from build123d import *

# Parameters (mm, degrees)
SKICA1_R                     = 15
P_IDAT_VYSUNUT_M1_DEPTH      = 2.5
SKICA1_3_R                   = 15
P_IDAT_VYSUNUT_M2_DEPTH      = 25
P_IDAT_VYSUNUT_M2_DEPTH_BACK = 5


with BuildPart() as part:
    # Skica1 → P_idat vysunut_m1 (new body, symmetric)
    with BuildSketch(Plane.XY):
        with BuildLine():
            Line((5, 30.562589032), (5, 5))
            Line((5, 5), (32.5, 5))
            Line((32.5, 5), (32.5, -5))
            Line((32.5, -5), (-32.5, -5))
            Line((-32.5, -5), (-32.5, 5))
            Line((-32.5, 5), (-5, 5))
            Line((-5, 5), (-5, 30.562589032))
            ThreePointArc((-5, 30.562589032), (0, 75), (5, 30.562589032))
        make_face()
        with Locations((0, 52.5)):
            Circle(SKICA1_R, mode=Mode.SUBTRACT)
        with BuildLine():
            Line((-5, 5), (-5, 30.562589032))
            ThreePointArc((-5, 30.562589032), (-22.358910385, 55.015775508), (-7.9e-08, 75))
            ThreePointArc((-7.9e-08, 75), (-16.889755219, 68.431933394), (-24.904867452, 52.178893569))
            Line((-24.904867452, 52.178893569), (-29.032485797, 5))
            Line((-29.032485797, 5), (-5, 5))
        make_face()
        with BuildLine():
            ThreePointArc((24.904867452, 52.178893569), (16.889755161, 68.431933447), (-7.9e-08, 75))
            ThreePointArc((-7.9e-08, 75), (22.358910376, 55.015775587), (5, 30.562589032))
            Line((5, 30.562589032), (5, 5))
            Line((5, 5), (29.032485797, 5))
            Line((29.032485797, 5), (24.904867452, 52.178893569))
        make_face()
    extrude(amount=P_IDAT_VYSUNUT_M1_DEPTH, both=True)

    # Skica1_3 → P_idat vysunut_m2 (add, two sides)
    with BuildSketch(Plane.XY) as p_idat_vysunut_m2_sk:
        with BuildLine():
            Line((5, 30.562589032), (5, 5))
            Line((5, 5), (32.5, 5))
            Line((32.5, 5), (32.5, -5))
            Line((32.5, -5), (-32.5, -5))
            Line((-32.5, -5), (-32.5, 5))
            Line((-32.5, 5), (-5, 5))
            Line((-5, 5), (-5, 30.562589032))
            ThreePointArc((-5, 30.562589032), (0, 75), (5, 30.562589032))
        make_face()
        with Locations((0, 52.5)):
            Circle(SKICA1_3_R, mode=Mode.SUBTRACT)
    extrude(amount=P_IDAT_VYSUNUT_M2_DEPTH)
    extrude(p_idat_vysunut_m2_sk.sketch, amount=-P_IDAT_VYSUNUT_M2_DEPTH_BACK)


solid = part.part
Check sheet for the modelled part. Datum: model origin and axes. Units: mm. A direction names the side the tool comes from. Give positions to 0.01 mm unless a question says otherwise; leave off trailing zeros. Write each loop counter-clockwise with the first axis right and the second up, starting at its lowest first coordinate (ties: lowest second). Pieces come first, ordered by that corner, then holes. Notation, with made-up numbers: (-8, 17) -> (30, 17) arc R13 cw to (30, 42) -> close; hole circle Ø4 at (-10, 18.5). An arc over 180 degrees is marked (long way). One line per item, written item: value. Start each with the question number.
Item 1: Material ranges on probe 1 along Y at (x, z) = (0, 10.5); probe 2 along Y at (x, z) = (10, -3.5); probe 3 along Z at (x, y) = (-7, 17.5), recorded low to high. Write a range as from..to.
Item 2: Section check D-D on x = 24. Record the cut outline in (y, z), then the cut area to 3 significant figures.
Item 3: Draft check along Y on faces 5 (the flat face through (0, -5, 10)), 6 (the flat face through (18, 25, -2.5)), 7 (the flat face through (-32.5, 0, 10)). Enter one of: +Y half, -Y half, draft (parallel to the pull), parting line (faces both ways), or undercut.
Item 4: Tool access check on faces 1 (the flat face through (5, 18, 14)), 2 (the cylindrical face through (-0.92, 74.98, 13.59)), 3 (the cylindrical face through (-0.92, 74.98, -3.73)), 4 (the flat face through (-18, 25, -2.5)). Record the directions out of +Z, -Z, +X, -X, +Y, -Y that give a thin tool (end or side, any length) a straight path to the whole face; none if there is none.
Item 5: Section check C-C on y = 63.5. Record the cut outline in (x, z), then the cut area to 3 significant figures.
Item 6: Section check A-A on z = 4.5. Record the cut outline in (x, y), then the cut area to 3 significant figures.
Item 7: Gauge pin test, flat ends, axial feed: pin 1 (0.8 mm diameter, centred on y = 19.5, z = -3.5, fed in from -X); pin 2 (10 mm diameter, centred on x = 8.5, z = -1.5, fed in from +Y); pin 3 (2 mm diameter, centred on y = 43, z = 17.5, fed in from -X); pin 4 (24 mm diameter, centred on x = 0, y = 52.5, fed in from +Z). Record the tip position at first contact, or that the pin passes through.
Item 8: Section check B-B on x = -9.5. Record the cut outline in (y, z).
Results list:
1. probe 1: -5..37.5, 67.5..75
1. probe 2: -5..5, 32.34..41.32, 63.68..72.66
1. probe 3: -2.5..2.5
2. outline: (-5, -5) -> (5, -5) -> (5, -2.5) -> (57, -2.5) -> (57, 2.5) -> (5, 2.5) -> (5, 25) -> (-5, 25) -> close
2. area: 560 mm²
3. face 5: -Y half
3. face 6: undercut
3. face 7: draft
4. face 1: +Z, +X
4. face 2: +Z
4. face 3: -Z
4. face 4: -Z, -X
5. outline: (-21.04, -2.5) -> (-19.63, -2.5) -> (-19.63, -5) -> (-10.2, -5) -> (-10.2, 25) -> (-19.63, 25) -> (-19.63, 2.5) -> (-21.04, 2.5) -> close; (10.2, -5) -> (19.63, -5) -> (19.63, -2.5) -> (21.04, -2.5) -> (21.04, 2.5) -> (19.63, 2.5) -> (19.63, 25) -> (10.2, 25) -> close
5. area: 580 mm²
6. outline: (-32.5, -5) -> (32.5, -5) -> (32.5, 5) -> (5, 5) -> (5, 30.56) arc R22.5 ccw (long way) to (-5, 30.56) -> (-5, 5) -> (-32.5, 5) -> close; hole circle Ø30 at (0, 52.5)
6. area: 1,790 mm²
7. pin 1: x = -5
7. pin 2: y = 74.75
7. pin 3: x = -20.83
7. pin 4: through
8. outline: (-5, -5) -> (5, -5) -> (5, -2.5) -> (32.1, -2.5) -> (32.1, -5) -> (40.89, -5) -> (40.89, 25) -> (32.1, 25) -> (32.1, 2.5) -> (5, 2.5) -> (5, 25) -> (-5, 25) -> close; (64.11, -5) -> (72.9, -5) -> (72.9, -2.5) -> (73.12, -2.5) -> (73.12, 2.5) -> (72.9, 2.5) -> (72.9, 25) -> (64.11, 25) -> close
